from build123d import *

# Parameters (mm, degrees)
F0_W        = 9
F0_H        = 2.25
F1_DEPTH    = 180
F2_T1_DEPTH = 192.6338141032
F3_R        = 2
F4_R        = 1.9


# Not quite as in the source:
# - a fillet or chamfer that OpenCascade refuses, or shapes differently, is made with other operations: its cross-section is extruded or revolved along the edge and cut away or added


with BuildPart() as f1:
    # F0 (on Front) → F1 (new body)
    with BuildSketch(Plane.XZ):
        Polygon((1.5, -2.25), (1.5, 0), (-7.5, -1.5), (-7.5, -3.75), align=None)
        Polygon((7.5, -7.5), (7.5, 7.5), (1.5, 7.5), (1.5, 0), (1.5, -2.25), (1.5, -5.25), (1.5, -7.5), align=None)
        with Locations((-3, -6.375)):
            Rectangle(F0_W, F0_H)
    extrude(amount=-F1_DEPTH)

    # F2: fillet of radius 3 on 1 edges, made by hand

    # F2_s2 → F2_t1 (cut)
    with BuildSketch(Plane.XZ.offset(-186.3169070516)):
        with BuildLine():
            ThreePointArc((-5.0076165068, -1.0846027511), (-6.7056654696, -1.9947746893), (-7.5, -3.75))
            Line((-7.5, -3.75), (-7.5, -1.5))
            Line((-7.5, -1.5), (-5.0076165068, -1.0846027511))
        make_face()
    extrude(amount=F2_T1_DEPTH, mode=Mode.SUBTRACT)

    # F3
    f3_edges = [f1.edges().sort_by_distance(p)[0] for p in [
        (-7.5, 90, -7.5),
    ]]
    fillet(f3_edges, radius=F3_R)

    # F4
    f4_edges = [f1.edges().sort_by_distance(p)[0] for p in [
        (1.5, 90, 7.5),
        (7.5, 90, 7.5),
    ]]
    fillet(f4_edges, radius=F4_R)


solid = f1.part
Read the model definition and answer for the solid it produces. Units are mm, in the model's axes. A direction names the side the tool comes from. Give positions to 0.01 mm unless a question says otherwise; leave off trailing zeros. Write each loop counter-clockwise with the first axis right and the second up, starting at its lowest first coordinate (ties: lowest second). Pieces come first, ordered by that corner, then holes. Notation, with made-up numbers: (89, 16) - (128, 16) arc R21 cw to (128, 24) - close; hole circle Ø8 at (23, 16). An arc over 180 degrees is marked (long way). Return JSON: item names as keys, results as strings.
Q1. A cutting plane is placed at A-A, the plane x = -0.25. Determine the outline of the cut face in (y, z).
Reply:
{"outline": "(0, -7.5) - (180, -7.5) - (180, -5.25) - (0, -5.25) - close; (0, -2.54) - (180, -2.54) - (180, -0.29) - (0, -0.29) - close"}
Q2. A cutting plane is placed at C-C, the plane z = 2.5. Determine the outline of the cut face in (x, y).
Reply:
{"outline": "(1.5, 0) - (7.5, 0) - (7.5, 180) - (1.5, 180) - close"}
Q3. A cutting plane is placed at B-B, the plane y = 137. Determine the outline of the cut face in (x, z).
Reply:
{"outline": "(-7.5, -5.5) arc R2 ccw to (-5.5, -7.5) - (7.5, -7.5) - (7.5, 5.6) arc R1.9 ccw to (5.6, 7.5) - (3.4, 7.5) arc R1.9 ccw to (1.5, 5.6) - (1.5, 0) - (-5.01, -1.08) arc R3 ccw to (-7.5, -3.75) - (1.5, -2.25) - (1.5, -5.25) - (-7.5, -5.25) - close"}
Q4. Consider line 1 along X through (y, z) = (26, 2.5); line 2 along Z through (x, y) = (-2.25, 121) (3 decimals); line 3 along Z through (x, y) = (-4.5, 161). Determine where each line is inside the solid, lowest interval first. Write a range as [from, to].
Reply:
{"line 1": "[1.5, 7.5]", "line 2": "[-7.5, -5.25], [-2.875, -0.625]", "line 3": "[-7.5, -5.25], [-3.25, -1]"}
Q5. Given P1, Ø4.5, axis at x = -4.5, y = 75, coming from the +Z side (3 decimals); P2, Ø1.5, axis at x = 1, y = 98, coming from the +Z side; P3, Ø4.5, axis at y = 124.5, z = 3, coming from the -X side, each flat-ended and moving along its own axis, determine where each tip first touches the part or whether it passes through.
Reply:
{"P1": "z = -0.625", "P2": "z = 6.54", "P3": "x = 1.5"}
Q6. For faces 4 (the face through (-3, 89, -3)), 5 (the face through (-3, 89, -5.25)), 6 (the face through (1.5, 89, 3)), determine the directions among +Z, -Z, +X, -X, +Y, -Y from which every point of the face is accessible in a straight line to the end or side of a thin tool.
Reply:
{"face 4": "+Y, -Y", "face 5": "-X, +Y, -Y", "face 6": "+Z, -X, +Y, -Y"}
Q7. For a pull along X with two mould halves and no side action, classify faces 1 (the face through (1.5, 89, -4)), 2 (the face through (2, 0, -2)), 3 (the face through (7.5, 89, -1)) as released by +X, released by -X, zero draft, split by the parting line, or undercut.
Reply:
{"face 1": "undercut", "face 2": "zero draft", "face 3": "released by +X"}
